Can you work these out from the drawing? Everything is in mm from the part's minimum corner. A direction names the side the tool comes from. Coordinates: 2 decimals unless noted, no trailing zeros. Order: outer loops, then holes, each group sorted by start corner. A loop starts at its lowest first (then second) coordinate and runs counter-clockwise, first axis right, second up. Notation, with made-up numbers: (-4.75, 18) - (43.25, 18) arc R14 ccw to (43.25, 23) - close; hole circle Ø8 at (51, 52). An arc over 180 degrees is marked (long way). Answer as CSV lines item,"result". Start each with the question number.
Item 1: On a 3-axis mill with a long thin cutter (end or side, diameter ignored), from which of +Z, -Z, +X, -X, +Y, -Y can I reach the whole of each face in a straight line? I mean the marked faces 1, 2 and 3. Say none if no direction works.
Item 2: Imagine slicing it at D-D on y = 9.25. List the corners of the cut face in (x, z) for me, and give its area (3 significant figures).
Item 3: I need wall thicknesses on line 1 (Y direction, x = 6.5, z = 7.75); line 2 (Y direction, x = 16.5, z = 6); line 3 (X direction, y = 4.75, z = 1). Which ranges of each line are inside material? Lowest first, please.
Item 4: Imagine slicing it at A-A on y = 7. List the corners of the cut face in (x, z) for me, and give its area (3 significant figures).
Item 5: Imagine slicing it at C-C on z = 5.5. List the corners of the cut face in (x, y) for me, and give its area (3 significant figures).
Item 6: Imagine slicing it at B-B on x = 9.5. List the corners of the cut face in (y, z) for me, and give its area (3 significant figures).
Item 7: I'm going to push flat-ended pins straight in: pin 1 (0.8 mm diameter, centred on x = 15.5, z = 7.5, fed in from +Y); pin 2 (2 mm diameter, centred on x = 15, z = 6, fed in from -Y); pin 3 (1.5 mm diameter, centred on y = 7.5, z = 1, fed in from +X). Where does each tip first touch, or does it pass through?
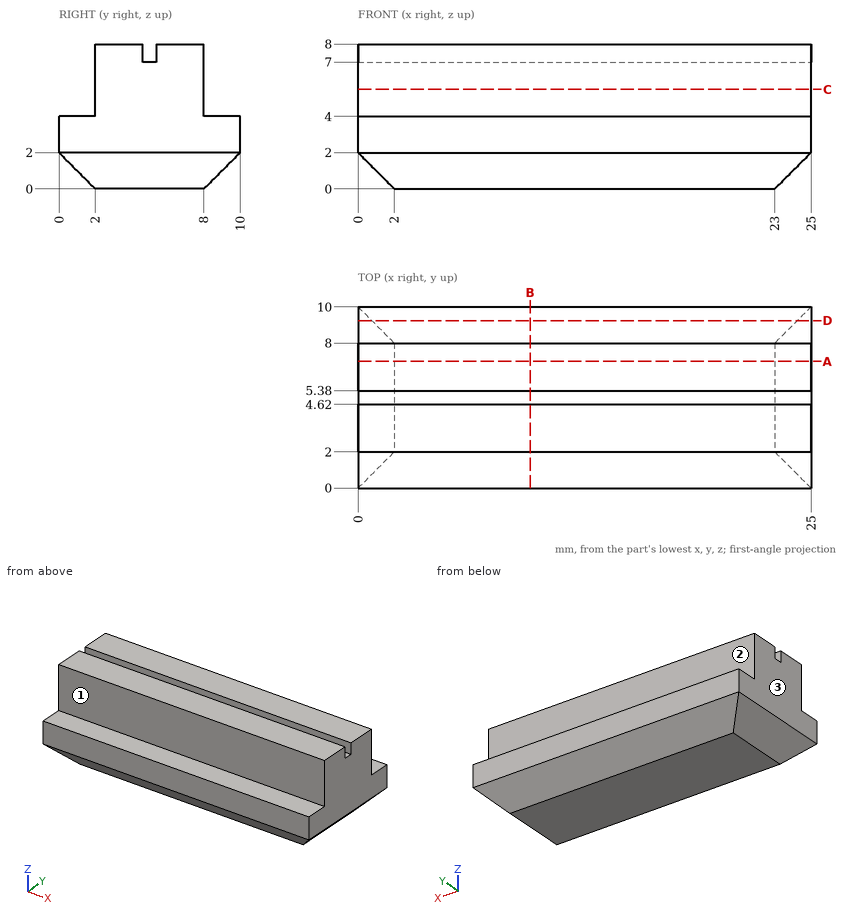
Responses:
1,face 1,"+Z, +X, -X, -Y"
1,face 2,"+Z, +X, -X, +Y"
1,face 3,"+Z, -Z, -X, +Y, -Y"
2,outline,"(0, 2) - (0.75, 1.25) - (24.25, 1.25) - (25, 2) - (25, 4) - (0, 4) - close"
2,area,"68.2 mm^2"
3,line 1,"y = 2 to 4.62, 5.38 to 8"
3,line 2,"y = 2 to 8"
3,line 3,"x = 1 to 24"
4,outline,"(0, 2) - (2, 0) - (23, 0) - (25, 2) - (25, 8) - (0, 8) - close"
4,area,"196 mm^2"
5,outline,"(0, 2) - (25, 2) - (25, 8) - (0, 8) - close"
5,area,"150 mm^2"
6,outline,"(0, 2) - (2, 0) - (8, 0) - (10, 2) - (10, 4) - (8, 4) - (8, 8) - (5.38, 8) - (5.38, 7) - (4.62, 7) - (4.62, 8) - (2, 8) - (2, 4) - (0, 4) - close"
6,area,"59.2 mm^2"
7,pin 1,"stops at y = 8"
7,pin 2,"stops at y = 2"
7,pin 3,"stops at x = 24.75"
